Work out the finished part from the listing and answer in its coordinate system (mm). A direction names the side the tool comes from. Give positions to 0.01 mm unless a question says otherwise; leave off trailing zeros. Order: outer loops, then holes, each group sorted by start corner. A loop starts at its lowest first (then second) coordinate and runs counter-clockwise, first axis right, second up. Notation, with made-up numbers: (23.5, 82.5) - (72.5, 82.5) arc R31 ccw to (72.5, 106.5) - close; hole circle Ø8 at (23.25, 41). An arc over 180 degrees is marked (long way). Return JSON: item names as keys, results as strings. Group by question number.
from build123d import *

# Parameters (mm, degrees)
SKETCH_R  = 1.7
SKETCH_W  = 21.5
SKETCH_H  = 13.6
PAD_DEPTH = 3.5
FILLET_R  = 1


with BuildPart() as part:
    # Sketch → Pad (new body)
    with BuildSketch(Plane.XY):
        with BuildLine():
            ThreePointArc((-20.921351, 17.61303), (-26.091433, 15.739591), (-26.413774, 10.249999))
            Line((-26.413774, 10.249999), (-4.330127, -28))
            ThreePointArc((-4.330127, -28), (0, -30.5), (4.330127, -28))
            Line((4.330127, -28), (26.413774, 10.249998))
            ThreePointArc((26.413774, 10.249998), (26.091434, 15.739591), (20.921351, 17.61303))
            ThreePointArc((-20.921351, 17.61303), (0, 15.147578), (20.921351, 17.61303))
        make_face()
        with Locations((-22.083648, 12.75)):
            Circle(SKETCH_R, mode=Mode.SUBTRACT)
        with Locations((22.083648, 12.75)):
            Circle(SKETCH_R, mode=Mode.SUBTRACT)
        with Locations((0, -25.5)):
            Circle(SKETCH_R, mode=Mode.SUBTRACT)
        Rectangle(SKETCH_W, SKETCH_H, mode=Mode.SUBTRACT)
    extrude(amount=PAD_DEPTH)

    # Fillet
    fillet_edges = [part.edges().sort_by_distance(p)[0] for p in [
        (-15.371951, -8.875001, 3.5),
        (-26.091433, 15.739591, 3.5),
        (0, 15.147578, 3.5),
        (26.091434, 15.739591, 3.5),
        (15.37195, -8.875001, 3.5),
        (0, -30.5, 3.5),
    ]]
    fillet(fillet_edges, radius=FILLET_R)


solid = part.part
1. The part is cut by section B-B (z = 0.6). Give the vertices of the cut face in (x, y).
2. The part is cut by section A-A (x = 0). Give the vertices of the cut face in (y, z).
3. The part is cut by section C-C (y = 12.75). State how many separate pieces and enclosed holes the cut face has, and give its area (3 significant figures).
4. A tool of negligible diameter and unlimited length cuts with its end or side. For faces 1 (the flat face through (0, 6.8, 2)), 2 (the cylindrical face through (-0.3, 15.15, 1.23)), from which of +Z, -Z, +X, -X, +Y, -Y can it reach the whole face along a straight path? Write none if from no direction.
5. Determine the mould class of faces 3 (the cylindrical face through (-0.221, -23.814, 1.726)), 4 (the flat face through (-15.527, -8.607, 1.232)), 5 (the cylindrical face through (-0.1, -30.5, 1.2)) for opening direction X: released by +X, released by -X, zero draft, split by the parting line, or undercut.
6. Each of these flat-tipped pins is pushed along its axis until it touches: pin 1 (1 mm diameter, centred on y = 2.5, z = 1, fed in from -X); pin 2 (1.8 mm diameter, centred on y = -1.5, z = 1, fed in from +X); pin 3 (4 mm diameter, centred on x = 22.08, y = 12.75, fed in from +Z); pin 4 (1 mm diameter, centred on x = 4.5, z = 2.5, fed in from -Y). Where does it stop, or does it pass through?
7. Consider probe 1 along X at (y, z) = (12.5, 0.95); probe 2 along Y at (x, z) = (23.5, 1.1); probe 3 along Y at (x, z) = (8, 2.2). Determine where each line is inside the solid, lowest interval first. Write a range as from..to.
Answers:
{
 "1": {"outline": "(-26.41, 10.25) - (-4.33, -28) arc R5 ccw to (4.33, -28) - (26.41, 10.25) arc R5 ccw to (20.92, 17.61) arc R90 cw to (-20.92, 17.61) arc R5 ccw to start; hole circle Ø3.4 at (-22.08, 12.75); hole (-10.75, -6.8) - (10.75, -6.8) - (10.75, 6.8) - (-10.75, 6.8) - close; hole circle Ø3.4 at (0, -25.5); hole circle Ø3.4 at (22.08, 12.75)"},
 "2": {"outline": "(-30.5, 0) - (-27.2, 0) - (-27.2, 3.5) - (-29.5, 3.5) arc R1 ccw to (-30.5, 2.5) - close; (-23.8, 0) - (-6.8, 0) - (-6.8, 3.5) - (-23.8, 3.5) - close; (6.8, 0) - (15.15, 0) - (15.15, 2.5) arc R1 ccw to (14.15, 3.5) - (6.8, 3.5) - close"},
 "3": {"separate pieces": "3", "enclosed holes": "0", "area": "165 mm^2"},
 "4": {"face 1": "+Z, -Z", "face 2": "+Z, -Z, +Y"},
 "5": {"face 3": "undercut", "face 4": "released by -X", "face 5": "split by the parting line"},
 "6": {"pin 1": "stops at x = -22.23", "pin 2": "stops at x = 20.15", "pin 3": "stops at z = 3.5", "pin 4": "stops at y = -28.5"},
 "7": {"probe 1": "x = -27.08..-23.77, -20.4..20.4, 23.77..27.08", "probe 2": "y = 5.2..11.81, 13.69..17.55", "probe 3": "y = -21.64..-6.8, 6.8..15.5"}
}
